from build123d import *

# Parameters (mm, degrees)
BOSS_EXTRUDE1_DEPTH = 15
SKETCH4_W           = 33.524511878
SKETCH4_H           = 20
CUT_EXTRUDE2_DEPTH  = 200


with BuildPart() as part:
    # Sketch1 → Boss-Extrude1 (new, symmetric)
    with BuildSketch(Plane(origin=(0, 0, 0), x_dir=(1, 0, 0), z_dir=(0, 1, 0))):
        with BuildLine():
            Line((-56.6451424, 1.085173475), (-53.646875163, 1.186754079))
            ThreePointArc((-53.646875163, 1.186754079), (1.186754079, 53.646875163), (53.646875163, -1.186754079))
            Line((53.646875163, -1.186754079), (56.645146911, -1.084937955))
            ThreePointArc((56.645146911, -1.084937955), (1.085055715, 56.645144656), (-56.6451424, 1.085173475))
        make_face()
    extrude(amount=BOSS_EXTRUDE1_DEPTH, both=True)

    # Sketch4 → Cut-Extrude2 (cut)
    with BuildSketch(Plane.XY):
        with Locations((-36.737744061, 0)):
            Rectangle(SKETCH4_W, SKETCH4_H)
        with Locations((36.737744061, 0)):
            Rectangle(SKETCH4_W, SKETCH4_H)
    extrude(amount=-CUT_EXTRUDE2_DEPTH, mode=Mode.SUBTRACT)


solid = part.part
The model under review builds one solid part; all positions refer to its coordinate system, in mm. A direction names the side the tool comes from. Round coordinates to 2 decimals unless told otherwise and drop trailing zeros. Write each loop counter-clockwise with the first axis right and the second up, starting at its lowest first coordinate (ties: lowest second). Pieces come first, ordered by that corner, then holes. Notation, with made-up numbers: M -29.75,-22.75 L -13.75,-22.75 A13 ccw -13.75,-5.75 Z; hole C -11,73 d10. An arc over 180 degrees is marked long. Use a Markdown table: item, result. Add a question column.
Q1. Insertion check: pin 1 (1 mm diameter, centred on y = -0.5, z = -51, fed in from -X); pin 2 (8 mm diameter, centred on x = -5.5, y = -12, fed in from +Z); pin 3 (12 mm diameter, centred on y = -3.5, z = -48, fed in from +X). Each pin has a flat end and moves straight along its axis. Give the tip position at first contact, or say it passes through.
Q2. We need section B-B, the plane z = -25. State the section outline as (x, y) points.
Q3. Machinability: for faces 1 (the face through (-53.5, 0, -11)), 2 (the face through (-19.975, 0, -51)), 3 (the face through (19.975, 0, -51)), which of the approach directions +Z, -Z, +X, -X, +Y, -Y give a long, thin tool a straight path to every point of the face, cutting with its end or side? Answer none if there is none.
Q4. We need section C-C, the plane x = 33.5. State the section outline as (y, z) points, plus the area to 3 significant figures.
Q5. We need section A-A, the plane y = 3.75. State the section outline as (x, z) points, plus the area to 3 significant figures.
Q6. The part is to be moulded in two halves that separate along Y. For faces 4 (the face through (-41, 10, -36)), 5 (the face through (4, 15, -54)), 6 (the face through (4, -15, -54)), say which applies: pulls with the +Y half, pulls with the -Y half, needs draft (parallel to the pull), parting line crosses it, or undercut.
Q7. To check wall thickness, follow line 1 (X direction, y = 12.75, z = -8.5); line 2 (X direction, y = 13.5, z = -4.5); line 3 (Z direction, x = -17.5, y = 2.75). State the ranges of each line that lie inside material, in increasing order.
Q8. We need section D-D, the plane z = -10. State the section outline as (x, y) points.
Findings below:
| question | item | result |
|---|---|---|
| 1 | pin 1 | stops at x = -19.98 |
| 1 | pin 2 | stops at z = -52.81 |
| 1 | pin 3 | stops at x = 19.98 |
| 2 | outline | M -50.84,-15 L -47.48,-15 L -47.48,-10 L -50.84,-10 Z; M -50.84,10 L -47.48,10 L -47.48,15 L -50.84,15 Z; M 47.48,-15 L 50.84,-15 L 50.84,-10 L 47.48,-10 Z; M 47.48,10 L 50.84,10 L 50.84,15 L 47.48,15 Z |
| 3 | face 1 | +Z, -Z |
| 3 | face 2 | +Z, -Z, -X |
| 3 | face 3 | +Z, -Z, +X |
| 4 | outline | M -15,-45.69 L -10,-45.69 L -10,-41.92 L -15,-41.92 Z; M 10,-45.69 L 15,-45.69 L 15,-41.92 L 10,-41.92 Z |
| 4 | area | 37.7 mm² |
| 5 | outline | M -56.65,-1.09 A56.66 ccw -53.5,-18.64 L -53.5,-4.14 A53.66 cw -53.65,-1.19 Z; M -19.98,-53.02 A56.66 ccw 19.98,-53.02 L 19.98,-49.8 A53.66 cw -19.98,-49.8 Z; M 53.5,-18.64 A56.66 ccw 56.65,1.08 L 53.65,1.19 A53.66 cw 53.5,-4.14 Z |
| 5 | area | 200 mm² |
| 6 | face 4 | undercut |
| 6 | face 5 | pulls with the +Y half |
| 6 | face 6 | pulls with the -Y half |
| 7 | line 1 | x = -56.01 to -52.98, 52.98 to 56.01 |
| 7 | line 2 | x = -56.48 to -53.47, 53.47 to 56.48 |
| 7 | line 3 | z = -53.89 to -50.73 |
| 8 | outline | M -55.77,-15 L -52.72,-15 L -52.72,-10 L -53.5,-10 L -53.5,10 L -52.72,10 L -52.72,15 L -55.77,15 Z; M 52.72,-15 L 55.77,-15 L 55.77,15 L 52.72,15 L 52.72,10 L 53.5,10 L 53.5,-10 L 52.72,-10 Z |
